Here's how the part is built. I have some questions about the finished solid (model axes, mm). Coordinates: 2 decimals unless noted, no trailing zeros. Loops run counter-clockwise (first coordinate to the right, second up) from the corner with the lowest first, then second, coordinate; pieces in that order, holes last. Notation, with made-up numbers: (65.5, 36) -> (124.5, 36) arc R19 cw to (124.5, 65) -> close; hole circle Ø7 at (22, 52.25). An arc over 180 degrees is marked (long way). Answer as a JSON object with one key per item and string values. Group by question number.
Q1. I need wall thicknesses on line 1 (X direction, y = 0.9, z = 70.5); line 2 (Z direction, x = 63.5, y = 1.55); line 3 (X direction, y = 0.6, z = 0). Which ranges of each line are inside material? Lowest first, please.
Q2. I want a section at B-B on z = 70.5. Write out the boundary of the cut face in (x, y).
Q3. I want a section at C-C on x = 0. Write out the boundary of the cut face in (y, z), then the cut area to 3 significant figures.
Q4. I want a section at A-A on x = 63.5. Write out the boundary of the cut face in (y, z), then the cut area to 3 significant figures.
Q5. Thinking about a two-plate mould opening in X: for faces 1 (the cylindrical face through (0.165, 1.05, -3.746)), 2 (the flat face through (15, 2.13, -1)), which applies, released by +X, released by -X, zero draft, split by the parting line, or undercut?
```python
from build123d import *

# Parameters (mm, degrees)
SKETCH1_W           = 140.3
SKETCH1_H           = 154.3
BOSS_EXTRUDE1_DEPTH = 2.13
SKETCH2_R           = 1.94
CUT_EXTRUDE1_DEPTH  = 31.13
SKETCH3_R           = 3.75
CUT_EXTRUDE2_DEPTH  = 20


with BuildPart() as part:
    # Sketch1 → Boss-Extrude1 (new body)
    with BuildSketch(Plane(origin=(0, 0, 0), x_dir=(1, 0, 0), z_dir=(0, 1, 0))):
        Rectangle(SKETCH1_W, SKETCH1_H)
    extrude(amount=BOSS_EXTRUDE1_DEPTH)

    # Sketch2 → Cut-Extrude1 (cut)
    with BuildSketch(Plane(origin=(0, 0, 0), x_dir=(1, 0, 0), z_dir=(0, 1, 0))):
        with Locations(Location((-63.5, -70.5, 0), (0, 0, 270))):
            Circle(SKETCH2_R)
        with Locations(Location((63.5, -70.5, 0), (0, 0, 270))):
            Circle(SKETCH2_R)
        with Locations(Location((-63.5, 70.5, 0), (0, 0, 270))):
            Circle(SKETCH2_R)
        with Locations(Location((63.5, 70.5, 0), (0, 0, 270))):
            Circle(SKETCH2_R)
    extrude(amount=CUT_EXTRUDE1_DEPTH, mode=Mode.SUBTRACT)

    # Sketch3 → Cut-Extrude2 (cut)
    with BuildSketch(Plane(origin=(0, 0, 0), x_dir=(1, 0, 0), z_dir=(0, 1, 0))):
        with Locations(Location((0, 0, 0), (0, 0, 270))):
            Circle(SKETCH3_R)
    extrude(amount=CUT_EXTRUDE2_DEPTH, mode=Mode.SUBTRACT)


solid = part.part
```
Result set:
{
 "1": {"line 1": "x = -70.15 to -65.44, -61.56 to 61.56, 65.44 to 70.15", "line 2": "z = -77.15 to -72.44, -68.56 to 68.56, 72.44 to 77.15", "line 3": "x = -70.15 to -3.75, 3.75 to 70.15"},
 "2": {"outline": "(-70.15, 0) -> (-65.44, 0) -> (-65.44, 2.13) -> (-70.15, 2.13) -> close; (-61.56, 0) -> (61.56, 0) -> (61.56, 2.13) -> (-61.56, 2.13) -> close; (65.44, 0) -> (70.15, 0) -> (70.15, 2.13) -> (65.44, 2.13) -> close"},
 "3": {"outline": "(0, -77.15) -> (2.13, -77.15) -> (2.13, -3.75) -> (0, -3.75) -> close; (0, 3.75) -> (2.13, 3.75) -> (2.13, 77.15) -> (0, 77.15) -> close", "area": "313 mm²"},
 "4": {"outline": "(0, -77.15) -> (2.13, -77.15) -> (2.13, -72.44) -> (0, -72.44) -> close; (0, -68.56) -> (2.13, -68.56) -> (2.13, 68.56) -> (0, 68.56) -> close; (0, 72.44) -> (2.13, 72.44) -> (2.13, 77.15) -> (0, 77.15) -> close", "area": "312 mm²"},
 "5": {"face 1": "undercut", "face 2": "zero draft"}
}
